Model file for the job. Use its own axes, mm. Face numbers are marked on the shaded views. A direction names the side the tool comes from. Round coordinates to 2 decimals unless told otherwise and drop trailing zeros. Write each loop counter-clockwise with the first axis right and the second up, starting at its lowest first coordinate (ties: lowest second). Pieces come first, ordered by that corner, then holes. Notation, with made-up numbers: (75, -28.75) - (97, -28.75) arc R21 ccw to (97, 7.25) - close; hole circle Ø8 at (31.25, 80.25). An arc over 180 degrees is marked (long way). Answer as a JSON object with one key per item and string values. Group by question number.
from build123d import *

# Parameters (mm, degrees)
SKETCH1_R           = 2.5
BOSS_EXTRUDE1_DEPTH = 80
SKETCH2_W           = 8
SKETCH2_H           = 8
BOSS_EXTRUDE2_DEPTH = 8
SKETCH3_R           = 2.5
BOSS_EXTRUDE3_DEPTH = 30


with BuildPart() as part:
    # Sketch1 → Boss-Extrude1 (new body)
    with BuildSketch(Plane(origin=(0, 0, 0), x_dir=(1, 0, 0), z_dir=(0, 1, 0))):
        Circle(SKETCH1_R)
    extrude(amount=BOSS_EXTRUDE1_DEPTH)

    # Sketch2 → Boss-Extrude2 (add)
    with BuildSketch(Plane(origin=(0, 80, 0), x_dir=(1, 0, 0), z_dir=(0, 1, 0))):
        Rectangle(SKETCH2_W, SKETCH2_H)
    extrude(amount=BOSS_EXTRUDE2_DEPTH)

    # Sketch3 → Boss-Extrude3 (add, symmetric)
    with BuildSketch(Plane(origin=(0, 0, 0), x_dir=(0, 0, -1), z_dir=(1, 0, 0))):
        with Locations((0, 84)):
            Circle(SKETCH3_R)
    extrude(amount=BOSS_EXTRUDE3_DEPTH, both=True)


solid = part.part
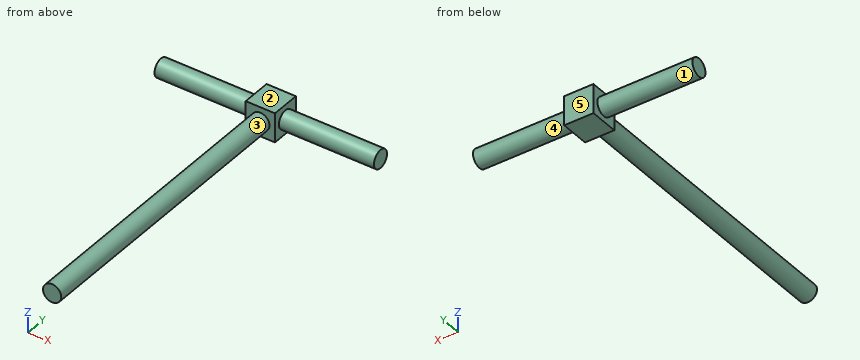
(1) Slice it at C-C (x = 1.5). Write the cut outline in (y, z).
(2) Slice it at D-D (x = 22). Write the cut outline in (y, z), then the cut area to 3 significant figures.
(3) Flat gauge pins, fed straight in: pin 1 (2 mm diameter, centred on x = -18, z = 1, fed in from -Y); pin 2 (8 mm diameter, centred on x = 4, y = 49, fed in from +Z); pin 3 (1 mm diameter, centred on x = 18.5, z = 0.5, fed in from +Y). Where does each tip first touch, or does it go through?
(4) Drill centre lines: line 1 (Z direction, x = 0, y = 45.5); line 2 (Y direction, x = -24, z = 0); line 3 (X direction, y = 31, z = -0.25). Where is each one in solid material? Low to high. Write a range as from..to.
(5) 3-axis set-ups, long thin cutter, end or side, ignore diameter. For the marked faces 1, 2, 3, 4 and 5: which of +Z, -Z, +X, -X, +Y, -Y reach the whole face in a straight line?
(6) Slice it at A-A (y = 84). Write the cut outline in (x, z).
(7) Slice it at B-B (z = 0). Write the cut outline in (x, y).
Answer:
{
 "1": {"outline": "(0, -2) - (80, -2) - (80, -4) - (88, -4) - (88, 4) - (80, 4) - (80, 2) - (0, 2) - close"},
 "2": {"outline": "circle Ø5 at (84, 0)", "area": "19.6 mm²"},
 "3": {"pin 1": "y = 81.5", "pin 2": "z = 2.5", "pin 3": "y = 86.5"},
 "4": {"line 1": "-2.5..2.5", "line 2": "81.5..86.5", "line 3": "-2.49..2.49"},
 "5": {"face 1": "-X", "face 2": "+Z, +X, -X, +Y, -Y", "face 3": "-Y", "face 4": "+X", "face 5": "+Z, -Z, +X, -X, +Y"},
 "6": {"outline": "(-30, -2.5) - (-4, -2.5) - (-4, -4) - (4, -4) - (4, -2.5) - (30, -2.5) - (30, 2.5) - (4, 2.5) - (4, 4) - (-4, 4) - (-4, 2.5) - (-30, 2.5) - close"},
 "7": {"outline": "(-30, 81.5) - (-4, 81.5) - (-4, 80) - (-2.5, 80) - (-2.5, 0) - (2.5, 0) - (2.5, 80) - (4, 80) - (4, 81.5) - (30, 81.5) - (30, 86.5) - (4, 86.5) - (4, 88) - (-4, 88) - (-4, 86.5) - (-30, 86.5) - close"}
}
